from build123d import *

# Parameters (mm, degrees)
F0_R     = 4.064
F1_DEPTH = 6.985
F2_R     = 1.27


with BuildPart() as f1:
    # F0 (on Top) → F1 (new body)
    with BuildSketch(Plane.XY):
        with BuildLine():
            ThreePointArc((-11.0109, 0), (-7.785882, 7.785882), (0, 11.0109))
            Line((0, 11.0109), (0, 18.796))
            ThreePointArc((0, 18.796), (-4.064, 22.86), (0, 26.924))
            Line((0, 26.924), (0, 31.115))
            Line((0, 31.115), (-22.86, 31.115))
            Line((-22.86, 31.115), (-22.86, 40.64))
            Line((-22.86, 40.64), (0, 40.64))
            Line((0, 40.64), (0, 45.72))
            Line((0, 45.72), (-33.02, 45.72))
            Line((-33.02, 45.72), (-33.02, 33.02))
            Line((-33.02, 33.02), (-45.72, 33.02))
            Line((-45.72, 33.02), (-45.72, 0))
            Line((-45.72, 0), (-40.64, 0))
            Line((-40.64, 0), (-40.64, 22.86))
            Line((-40.64, 22.86), (-31.115, 22.86))
            Line((-31.115, 22.86), (-31.115, 0))
            Line((-31.115, 0), (-26.924, 0))
            ThreePointArc((-26.924, 0), (-22.86, 4.064), (-18.796, 0))
            Line((-18.796, 0), (-11.0109, 0))
        make_face()
        with Locations((-16.164461, 16.164461)):
            Circle(F0_R, mode=Mode.SUBTRACT)
        with BuildLine():
            ThreePointArc((0, 11.0109), (7.785882, 7.785882), (11.0109, 0))
            Line((11.0109, 0), (18.796, 0))
            ThreePointArc((18.796, 0), (22.86, 4.064), (26.924, 0))
            Line((26.924, 0), (31.115, 0))
            Line((31.115, 0), (31.115, 22.86))
            Line((31.115, 22.86), (40.64, 22.86))
            Line((40.64, 22.86), (40.64, 0))
            Line((40.64, 0), (45.72, 0))
            Line((45.72, 0), (45.72, 33.02))
            Line((45.72, 33.02), (33.02, 33.02))
            Line((33.02, 33.02), (33.02, 45.72))
            Line((33.02, 45.72), (0, 45.72))
            Line((0, 45.72), (0, 40.64))
            Line((0, 40.64), (22.86, 40.64))
            Line((22.86, 40.64), (22.86, 31.115))
            Line((22.86, 31.115), (0, 31.115))
            Line((0, 31.115), (0, 26.924))
            ThreePointArc((0, 26.924), (2.873682, 25.733682), (4.064, 22.86))
            ThreePointArc((4.064, 22.86), (2.873682, 19.986318), (0, 18.796))
            Line((0, 18.796), (0, 11.0109))
        make_face()
        with Locations((16.164461, 16.164461)):
            Circle(F0_R, mode=Mode.SUBTRACT)
        with BuildLine():
            Line((18.796, 0), (11.0109, 0))
            ThreePointArc((11.0109, 0), (7.785882, -7.785882), (0, -11.0109))
            Line((0, -11.0109), (0, -18.796))
            ThreePointArc((0, -18.796), (2.873682, -19.986318), (4.064, -22.86))
            ThreePointArc((4.064, -22.86), (2.873682, -25.733682), (0, -26.924))
            Line((0, -26.924), (0, -31.115))
            Line((0, -31.115), (22.86, -31.115))
            Line((22.86, -31.115), (22.86, -40.64))
            Line((22.86, -40.64), (0, -40.64))
            Line((0, -40.64), (0, -45.72))
            Line((0, -45.72), (33.02, -45.72))
            Line((33.02, -45.72), (33.02, -33.02))
            Line((33.02, -33.02), (45.72, -33.02))
            Line((45.72, -33.02), (45.72, 0))
            Line((45.72, 0), (40.64, 0))
            Line((40.64, 0), (40.64, -22.86))
            Line((40.64, -22.86), (31.115, -22.86))
            Line((31.115, -22.86), (31.115, 0))
            Line((31.115, 0), (26.924, 0))
            ThreePointArc((26.924, 0), (22.86, -4.064), (18.796, 0))
        make_face()
        with Locations((16.164461, -16.164461)):
            Circle(F0_R, mode=Mode.SUBTRACT)
        with BuildLine():
            Line((0, -18.796), (0, -11.0109))
            ThreePointArc((0, -11.0109), (-7.785882, -7.785882), (-11.0109, 0))
            Line((-11.0109, 0), (-18.796, 0))
            ThreePointArc((-18.796, 0), (-22.86, -4.064), (-26.924, 0))
            Line((-26.924, 0), (-31.115, 0))
            Line((-31.115, 0), (-31.115, -22.86))
            Line((-31.115, -22.86), (-40.64, -22.86))
            Line((-40.64, -22.86), (-40.64, 0))
            Line((-40.64, 0), (-45.72, 0))
            Line((-45.72, 0), (-45.72, -33.02))
            Line((-45.72, -33.02), (-33.02, -33.02))
            Line((-33.02, -33.02), (-33.02, -45.72))
            Line((-33.02, -45.72), (0, -45.72))
            Line((0, -45.72), (0, -40.64))
            Line((0, -40.64), (-22.86, -40.64))
            Line((-22.86, -40.64), (-22.86, -31.115))
            Line((-22.86, -31.115), (0, -31.115))
            Line((0, -31.115), (0, -26.924))
            ThreePointArc((0, -26.924), (-4.064, -22.86), (0, -18.796))
        make_face()
        with Locations((-16.164461, -16.164461)):
            Circle(F0_R, mode=Mode.SUBTRACT)
    extrude(amount=F1_DEPTH)

    # F2
    f2_edges = [f1.edges().sort_by_distance(p)[0] for p in [
        (0, 45.72, 6.985),
        (-33.02, 39.37, 6.985),
        (-39.37, 33.02, 6.985),
        (-45.72, 0, 6.985),
        (-33.02, -39.37, 6.985),
        (-39.37, -33.02, 6.985),
        (0, -45.72, 6.985),
        (33.02, -39.37, 6.985),
        (39.37, -33.02, 6.985),
        (45.72, 0, 6.985),
        (39.37, 33.02, 6.985),
        (33.02, 39.37, 6.985),
        (0, -45.72, 0),
        (-33.02, -39.37, 0),
        (-39.37, -33.02, 0),
        (-45.72, 0, 0),
        (-39.37, 33.02, 0),
        (-33.02, 39.37, 0),
        (0, 45.72, 0),
        (33.02, 39.37, 0),
        (39.37, 33.02, 0),
        (45.72, 0, 0),
        (39.37, -33.02, 0),
        (33.02, -39.37, 0),
    ]]
    fillet(f2_edges, radius=F2_R)


solid = f1.part
Read the model definition and answer for the solid it produces. Units are mm, in the model's axes. A direction names the side the tool comes from. Give positions to 0.01 mm unless a question says otherwise; leave off trailing zeros. Write each loop counter-clockwise with the first axis right and the second up, starting at its lowest first coordinate (ties: lowest second). Pieces come first, ordered by that corner, then holes. Notation, with made-up numbers: (52, -20) - (82, -20) arc R21 ccw to (82, 14) - close; hole circle Ø5 at (-17.5, -13). An arc over 180 degrees is marked (long way). Use CSV: the item, a comma, the result in double quotes. Start each with the question number.
(1) Find section C-C (y = 14). Give the vertices of the cut face in (x, z) (3 decimals).
(2) For faces 1 (the flat face through (-33.02, -39, 3)), 2 (the flat face through (40.64, 0, 3)), 3 (the flat face through (33.02, -39, 3)), 4 (the flat face through (0, 45.72, 3)), 5 (the flat face through (-11, 11, 0)), determine the directions among +Z, -Z, +X, -X, +Y, -Y from which every point of the face is accessible in a straight line to the end or side of a thin tool.
(3) Find section A-A (y = 38). Give the vertices of the cut face in (x, z) (3 decimals), plus the area to 3 significant figures.
(4) Find section B-B (x = 3). Give the vertices of the cut face in (y, z) (3 decimals).
(5) Find section D-D (z = 3.75). Count the separate pieces of the cut face and the enclosed holes in it, plus the area to 3 significant figures.
(6) Consider line 1 along X through (y, z) = (-16.5, 3) (3 decimals); line 2 along Y through (x, z) = (-12, 1.75) (3 decimals); line 3 along X through (y, z) = (35, 2.25). Determine where each line is inside the solid, lowest interval first.
(7) Given P1, Ø2, axis at y = 11.5, z = 1, coming from the +X side; P2, Ø2, axis at x = 40.5, z = 3.5, coming from the -Y side; P3, Ø1.3, axis at y = 40, z = 3, coming from the -X side; P4, Ø2, axis at x = -40.5, z = 3.5, coming from the +Y side, each flat-ended and moving along its own axis, determine where each tip first touches the part or whether it passes through.
Findings below:
1,outline,"(-45.72, 1.27) arc R1.27 ccw to (-44.45, 0) - (-40.64, 0) - (-40.64, 6.985) - (-44.45, 6.985) arc R1.27 ccw to (-45.72, 5.715) - close; (-31.115, 0) - (-19.604, 0) - (-19.604, 6.985) - (-31.115, 6.985) - close; (-12.725, 0) - (12.725, 0) - (12.725, 6.985) - (-12.725, 6.985) - close; (19.604, 0) - (31.115, 0) - (31.115, 6.985) - (19.604, 6.985) - close; (40.64, 0) - (44.45, 0) arc R1.27 ccw to (45.72, 1.27) - (45.72, 5.715) arc R1.27 ccw to (44.45, 6.985) - (40.64, 6.985) - close"
2,face 1,"+Z, -Z, -X, -Y"
2,face 2,"+Z, -Z"
2,face 3,"+Z, -Z, +X, -Y"
2,face 4,"+Z, -Z, +X, -X, +Y"
2,face 5,"-Z, +X, -X, +Y, -Y"
3,outline,"(-33.02, 1.27) arc R1.27 ccw to (-31.75, 0) - (-22.86, 0) - (-22.86, 6.985) - (-31.75, 6.985) arc R1.27 ccw to (-33.02, 5.715) - close; (22.86, 0) - (31.75, 0) arc R1.27 ccw to (33.02, 1.27) - (33.02, 5.715) arc R1.27 ccw to (31.75, 6.985) - (22.86, 6.985) - close"
3,area,"141 mm2"
4,outline,"(-45.72, 1.27) arc R1.27 ccw to (-44.45, 0) - (-40.64, 0) - (-40.64, 6.985) - (-44.45, 6.985) arc R1.27 ccw to (-45.72, 5.715) - close; (-31.115, 0) - (-25.602, 0) - (-25.602, 6.985) - (-31.115, 6.985) - close; (-20.118, 0) - (-10.594, 0) - (-10.594, 6.985) - (-20.118, 6.985) - close; (10.594, 0) - (20.118, 0) - (20.118, 6.985) - (10.594, 6.985) - close; (25.602, 0) - (31.115, 0) - (31.115, 6.985) - (25.602, 6.985) - close; (40.64, 0) - (44.45, 0) arc R1.27 ccw to (45.72, 1.27) - (45.72, 5.715) arc R1.27 ccw to (44.45, 6.985) - (40.64, 6.985) - close"
5,separate pieces,"1"
5,enclosed holes,"13"
5,area,"5,180 mm2"
6,line 1,"-45.72 to -40.64, -31.115 to -20.215, -12.114 to 12.114, 20.215 to 31.115, 40.64 to 45.72"
6,line 2,"-45.72 to -40.64, -31.115 to 31.115, 40.64 to 45.72"
6,line 3,"-33.02 to -22.86, 22.86 to 33.02"
7,P1,"x = 45.72"
7,P2,"y = -33.02"
7,P3,"x = -33.02"
7,P4,"y = 33.02"
